Answer from the drawing. Dimensions are ordinates in mm from the lowest x, y and z of the part. Give positions to 0.01 mm unless a question says otherwise; leave off trailing zeros. Order: outer loops, then holes, each group sorted by start corner. A loop starts at its lowest first (then second) coordinate and runs counter-clockwise, first axis right, second up. Notation, with made-up numbers: (16.5, 86.25) - (39.5, 86.25) arc R17 cw to (39.5, 93.25) - close; hole circle Ø4 at (5, 42.25). An arc over 180 degrees is marked (long way). Use a Markdown table: item, result. Add a question column.
1) Find section C-C, the plane z = 8. Determine the outline of the cut face in (x, y), plus the area to 3 significant figures.
2) Find section D-D, the plane y = 1.5. Determine the outline of the cut face in (x, z).
3) Find section A-A, the plane x = 25. Determine the outline of the cut face in (y, z), plus the area to 3 significant figures.
4) Find section B-B, the plane z = 87. Determine the outline of the cut face in (x, y), plus the area to 3 significant figures.
5) A flat-ended cylindrical pin translates along its axis: pin 1 (4 mm diameter, centred on x = 50, y = 5, fed in from +Z). Find the tip coordinate at first contact, or state that the pin passes through.
6) Straight lines are drawn through the part: line 1 (Z direction, x = 80, y = 2); line 2 (Z direction, x = 8, y = 4.75); line 3 (Y direction, x = 50, z = 129). For each, find the intervals that lie inside material, in ascending order.
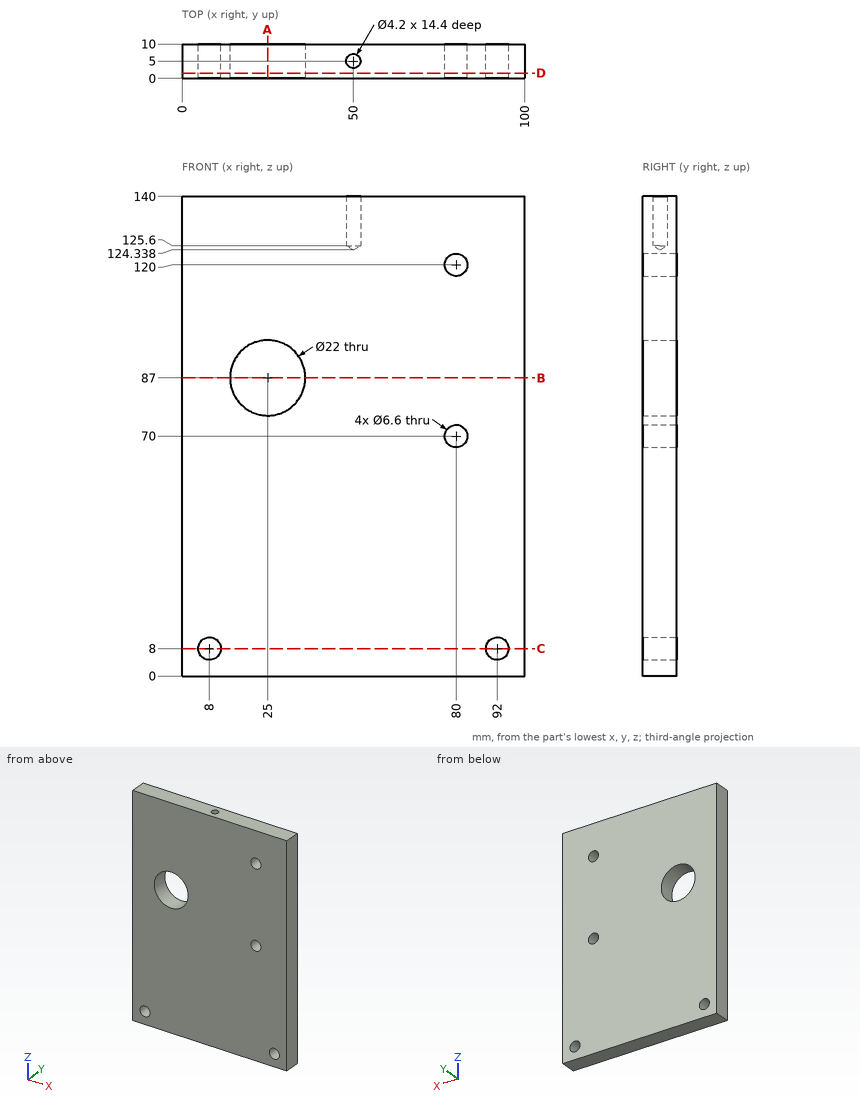
The answers:
| question | item | result |
|---|---|---|
| 1 | outline | (0, 0) - (4.7, 0) - (4.7, 10) - (0, 10) - close; (11.3, 0) - (88.7, 0) - (88.7, 10) - (11.3, 10) - close; (95.3, 0) - (100, 0) - (100, 10) - (95.3, 10) - close |
| 1 | area | 868 mm2 |
| 2 | outline | (0, 0) - (100, 0) - (100, 140) - (0, 140) - close; hole circle Ø6.6 at (8, 8); hole circle Ø22 at (25, 87); hole circle Ø6.6 at (80, 70); hole circle Ø6.6 at (80, 120); hole circle Ø6.6 at (92, 8) |
| 3 | outline | (0, 0) - (10, 0) - (10, 76) - (0, 76) - close; (0, 98) - (10, 98) - (10, 140) - (0, 140) - close |
| 3 | area | 1,180 mm2 |
| 4 | outline | (0, 0) - (14, 0) - (14, 10) - (0, 10) - close; (36, 0) - (100, 0) - (100, 10) - (36, 10) - close |
| 4 | area | 780 mm2 |
| 5 | pin 1 | z = 125.54 |
| 6 | line 1 | 0 to 66.7, 73.3 to 116.7, 123.3 to 140 |
| 6 | line 2 | 0 to 4.7, 11.3 to 140 |
| 6 | line 3 | 0 to 2.9, 7.1 to 10 |
